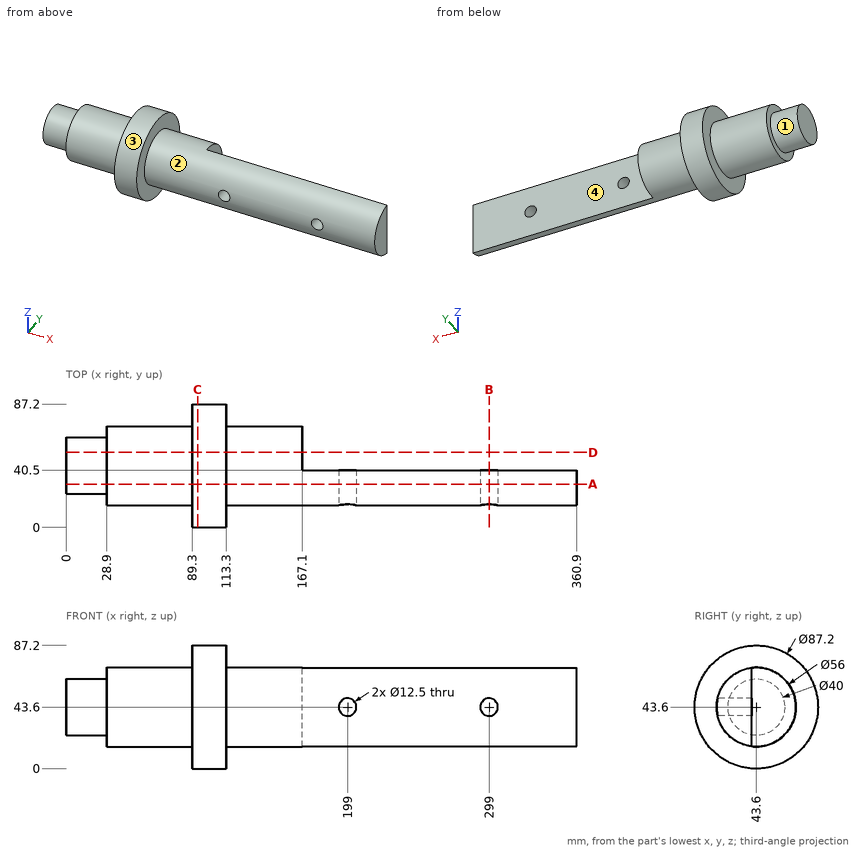
Geometry: see drawing. Coordinates: mm, zero at the bounding-box minimum. A direction names the side the tool comes from. Round coordinates to 2 decimals unless told otherwise and drop trailing zeros. Write each loop counter-clockwise with the first axis right and the second up, starting at its lowest first coordinate (ties: lowest second). Pieces come first, ordered by that corner, then holes. Notation, with made-up numbers: M -11.75,-9 L 4.25,-9 A17 cw 4.25,15 Z; hole C 47,-35 d10. An arc over 180 degrees is marked long. Answer as a JSON object with one key per item and string values. Group by question number.
(1) Section query A-A on y = 30.5. Output: boundary loops of the cut face in (x, z), then the cut area to 3 significant figures.
(2) Section query B-B on x = 299. Output: boundary loops of the cut face in (y, z), then the cut area to 3 significant figures.
(3) Section query D-D on y = 53. Output: boundary loops of the cut face in (x, z), then the cut area to 3 significant figures.
(4) First-contact query: pin 1 (4 mm diameter, centred on y = 13, z = 30, fed in from -X); pin 2 (2 mm diameter, centred on y = 60.5, z = 24.5, fed in from +X); pin 3 (6 mm diameter, centred on x = 323.5, y = 40, fed in from -Z). Flat tips, straight axial feed; report the tip coordinate or a pass-through.
(5) Section query C-C on x = 93. Output: boundary loops of the cut face in (y, z), then the cut area to 3 significant figures.
(6) Ray query, line 1 (X direction, y = 21, z = 43); line 2 (X direction, y = 27.5, z = 43.6); line 3 (Z direction, x = 199, y = 24). Return the intervals inside material, ascending. Write a range as [from, to].
(7) Reachability of the marked faces 1, 2, 3 and 4 from +Z, -Z, +X, -X, +Y, -Y: full face, straight path, thin tool, end or side. Return the list, or none.
Computed values:
{
 "1": {"outline": "M 0,28.49 L 28.9,28.49 L 28.9,18.85 L 89.3,18.85 L 89.3,2.01 L 113.3,2.01 L 113.3,18.85 L 360.9,18.85 L 360.9,68.35 L 113.3,68.35 L 113.3,85.19 L 89.3,85.19 L 89.3,68.35 L 28.9,68.35 L 28.9,58.71 L 0,58.71 Z; hole C 199,43.6 d12.5; hole C 299,43.6 d12.5", "area": "17,900 mm^2"},
 "2": {"outline": "M 16.31,37.35 A28 ccw 40.5,15.77 L 40.5,37.35 Z; M 16.31,49.85 L 40.5,49.85 L 40.5,71.43 A28 ccw Z", "area": "750 mm^2"},
 "3": {"outline": "M 0,25.95 L 28.9,25.95 L 28.9,17.23 L 89.3,17.23 L 89.3,1.03 L 113.3,1.03 L 113.3,17.23 L 167.1,17.23 L 167.1,69.97 L 113.3,69.97 L 113.3,86.17 L 89.3,86.17 L 89.3,69.97 L 28.9,69.97 L 28.9,61.25 L 0,61.25 Z", "area": "9,090 mm^2"},
 "4": {"pin 1": "x = 89.3", "pin 2": "x = 167.1", "pin 3": "z = 15.77"},
 "5": {"outline": "C 43.6,43.6 d87.2", "area": "5,970 mm^2"},
 "6": {"line 1": "[28.9, 192.78], [205.22, 292.78], [305.22, 360.9]", "line 2": "[0, 192.75], [205.25, 292.75], [305.25, 360.9]", "line 3": "[23.6, 37.35], [49.85, 63.6]"},
 "7": {"face 1": "-X", "face 2": "+X", "face 3": "+X, -X", "face 4": "+Z, -Z, +X, +Y"}
}
